Work out the finished part from the listing and answer in its coordinate system (mm). Coordinates: 2 decimals unless noted, no trailing zeros. Order: outer loops, then holes, each group sorted by start corner. A loop starts at its lowest first (then second) coordinate and runs counter-clockwise, first axis right, second up. Notation, with made-up numbers: M 17.5,85 L 33.5,85 A30 cw 33.5,107 Z; hole C 1,44.25 d1. An arc over 180 degrees is marked long. Use a Markdown table: item, result.
from build123d import *

# Parameters (mm, degrees)
SKETCH1_R          = 3
EXTRUDE1_DEPTH     = 100
CHAMFER1_SIZE      = 0.6
SKETCH3_R          = 10.435428451
CUT_EXTRUDE1_DEPTH = 100


with BuildPart() as part:
    # Sketch1 → Extrude1 (new, symmetric)
    with BuildSketch(Plane.XY):
        Circle(SKETCH1_R)
    extrude(amount=EXTRUDE1_DEPTH, both=True)

    # Chamfer1
    chamfer1_edges = [part.edges().sort_by_distance(p)[0] for p in [
        (-3, 0, -100),
        (-3, 0, 100),
    ]]
    chamfer(chamfer1_edges, length=CHAMFER1_SIZE)

    # Sketch3 → Cut-Extrude1 (cut)
    with BuildSketch(Plane.XY.offset(100)):
        Circle(SKETCH3_R)
    extrude(amount=-CUT_EXTRUDE1_DEPTH, mode=Mode.SUBTRACT)


solid = part.part
(1) A cutting plane is placed at A-A (z = -45.5). Determine the outline of the cut face in (x, y), then the cut area to 3 significant figures.
Conclusion:
| item | result |
|---|---|
| outline | C 0,0 d6 |
| area | 28.3 mm2 |
(2) Given P1, Ø2, axis at y = -1.5, z = -16.5, coming from the -X side; P2, Ø1.5, axis at y = -2, z = -66, coming from the +X side; P3, Ø3, axis at x = 1.5, z = -43.5, coming from the -Y side, each flat-ended and moving along its own axis, determine where each tip first touches the part or whether it passes through.
Conclusion:
| item | result |
|---|---|
| P1 | x = -2.96 |
| P2 | x = 2.73 |
| P3 | y = -3 |
(3) Straight lines are drawn through the part: L1, parallel to X at y = -0.35, z = -46.5; L2, parallel to Y at x = -0.25, z = -44; L3, parallel to Y at x = 2.5, z = -50. For each, find the intervals that lie inside material, in ascending order.
Conclusion:
| item | result |
|---|---|
| L1 | -2.98 to 2.98 |
| L2 | -2.99 to 2.99 |
| L3 | -1.66 to 1.66 |
